Check sheet for the modelled part. Datum: model origin and axes. Units: mm. A direction names the side the tool comes from. Round coordinates to 2 decimals unless told otherwise and drop trailing zeros. Write each loop counter-clockwise with the first axis right and the second up, starting at its lowest first coordinate (ties: lowest second). Pieces come first, ordered by that corner, then holes. Notation, with made-up numbers: M -9.75,-24.5 L 21.25,-24.5 A21 cw 21.25,13.5 Z; hole C -29,-30 d10. An arc over 180 degrees is marked long. Put each result on its own line as item: value.
Autodesk Inventor part; units mm, degrees
ref_plane "YZ Plane" through (0, 0, 0) normal (1, 0, 0) x (0, 1, 0)
ref_plane "XZ Plane" through (0, 0, 0) normal (0, 1, 0) x (-1, 0, 0)
ref_plane "XY Plane" through (0, 0, 0) normal (0, 0, 1) x (1, 0, 0)
sketch "スケッチ1" plane through (0, 0, 0) normal (0, 0, 1) x (1, 0, 0)
  circle A0 centre (0, 0) radius 3
  dimension "d0" = 6
extrude "押し出し1" add sketch "スケッチ1" along normal blind 10
sketch "スケッチ2" plane through (0, 0, 0) normal (0, 0, -1) x (-1, 0, 0)
  circle A0 centre (0, 0) radius 1.5
  dimension "d3" = 3
extrude "押し出し2" cut sketch "スケッチ2" against normal blind 1
sketch "スケッチ3" plane through (0, 0, 0) normal (1, 0, 0) x (0, 1, 0)
  line L0 (-3, 0) -> (-3, 10)
  line L1 (-3, 10) -> (3, 10)
  line L2 (3, 10) -> (3, 0)
  line L3 (3, 0) -> (1.5, 0)
  line L4 (1.5, 0) -> (1.5, 1)
  line L5 (1.5, 1) -> (-1.5, 1)
  line L6 (-1.5, 1) -> (-1.5, 0)
  line L7 (-1.5, 0) -> (-3, 0)
  arc A0 (-1.5, 1) -> (1.5, 1) centre (0, 1.625) ccw
  line L8 (0, 0) -> (0, 1)
revolve "回転1" add sketch "スケッチ3" angle 360 about axis through (0, 0, 0) along (0, 0, 1) picked at (0.9377, 0.8892) contours L5 A0 L8
sketch "スケッチ4" plane through (0, 0, 10) normal (0, 0, 1) x (1, 0, 0)
  circle A0 centre (0, 0) radius 3
  line L0 (1.5, 2.5981) -> (-1.5, 2.5981)
  line L1 (-1.5, 2.5981) -> (-1.5, -2.5981)
  line L2 (-1.5, -2.5981) -> (1.5, -2.5981)
  line L3 (1.5, -2.5981) -> (1.5, 2.5981)
  line L4 (1.5, 2.5981) -> (-1.5, -2.5981) construction
  line L5 (-1.5, 2.5981) -> (1.5, -2.5981) construction
  dimension "d7" = 3
extrude "押し出し3" add sketch "スケッチ4" along normal blind 8 contours L3 L2 L1 L0
fillet "フィレット1" radius 0.2 4 edges at (-1.5, -2.5981, 14) (1.5, -2.5981, 14) (-1.5, 2.5981, 14) (1.5, 2.5981, 14)
properties part number "FU650AD5-C6" material "ABS プラスチック"
1. Cross-section at A-A (x = 0). Enter the section's corners in (y, z) (3 decimals), then the cut area to 3 significant figures.
Computed values:
outline: M -3,0 L -1.5,0 L -1.5,1 A1.625 ccw 1.5,1 L 1.5,0 L 3,0 L 3,10 L 2.598,10 L 2.598,18 L -2.598,18 L -2.598,10 L -3,10 Z
area: 101 mm2
2. Depth check by flat-ended pin: pin 1 Ø1 at (y, z) = (1, 6.5) entering from -X; pin 2 Ø1.3 at (x, z) = (0, 13.5) entering from -Y; pin 3 Ø2 at (x, z) = (0.5, 12.5) entering from +Y. Enter the tip coordinate at first touch or a pass-through.
Computed values:
pin 1: stops at x = -2.96
pin 2: stops at y = -2.6
pin 3: stops at y = 2.6
3. Cross-section at B-B (y = -0.25). Enter the section's corners in (x, z) (3 decimals), then the cut area to 3 significant figures.
Computed values:
outline: M -2.99,0 L -1.479,0 L -1.479,1 A1.606 ccw 1.479,1 L 1.479,0 L 2.99,0 L 2.99,10 L 1.5,10 L 1.5,18 L -1.5,18 L -1.5,10 L -2.99,10 Z
area: 82.9 mm2
4. Cross-section at D-D (y = -2). Enter the section's corners in (x, z).
Computed values:
outline: M -2.24,0 L 2.24,0 L 2.24,10 L 1.5,10 L 1.5,18 L -1.5,18 L -1.5,10 L -2.24,10 Z
5. Scan lines: probe 1 along Y at (x, z) = (0, 0.65); probe 2 along X at (y, z) = (0, 0.35); probe 3 along X at (y, z) = (0, 0.3). Record each from-to range of solid material in increasing order.
Computed values:
probe 1: y = -3 to -1.5, -1.3 to 1.3, 1.5 to 3
probe 2: x = -3 to -1.5, -1.01 to 1.01, 1.5 to 3
probe 3: x = -3 to -1.5, -0.94 to 0.94, 1.5 to 3
6. Access from +Z, -Z, +X, -X, +Y, -Y to the whole of each face (thin tool, end or side, straight path). Record for faces 1 (the flat face through (0, -2.598, 14)), 2 (the flat face through (0, 2.598, 14)), 3 (the flat face through (-1.5, 0, 14)).
Computed values:
face 1: +Z, +X, -X, -Y
face 2: +Z, +X, -X, +Y
face 3: +Z, -X, +Y, -Y
7. Cross-section at C-C (z = 8.25). Enter the section's corners in (x, y), then the cut area to 3 significant figures.
Computed values:
outline: C 0,0 d6
area: 28.3 mm2
